from build123d import *

# Parameters (mm, degrees)
SKETCH1_R          = 10
SKETCH1_R_2        = 2.5
SKETCH1_R_3        = 15
SKETCH1_R_4        = 5
BASE_FLANGE1_DEPTH = 3.4


# Sheet-metal steps are written as plain solids
with BuildPart() as part:
    # Sketch1 → Base-Flange1 (new body)
    with BuildSketch(Plane.XY):
        Polygon((0, 63.731432889), (0, 0), (-95.246303627, 0), (-424.746303627, 118), (-484.746303627, 118), (-594.746303627, 58), (-654.746303627, 58), (-654.746303627, 118), (-594.746303627, 118), (-484.746303627, 181.731432889), (-424.746303627, 181.731432889), (-95.246303627, 63.731432889), align=None)
        with Locations((-624.746303627, 88)):
            Circle(SKETCH1_R, mode=Mode.SUBTRACT)
        with Locations((-454.746303627, 149.865716445)):
            Circle(SKETCH1_R, mode=Mode.SUBTRACT)
        with Locations((-539.746303627, 118.932858222)):
            Circle(SKETCH1_R_2, mode=Mode.SUBTRACT)
        with Locations((-161.147850314, 55.466270342)):
            Circle(SKETCH1_R_3, mode=Mode.SUBTRACT)
        with Locations((-255.29291701, 89.181347338)):
            Circle(SKETCH1_R_2, mode=Mode.SUBTRACT)
        with Locations((-349.437983706, 122.896424333)):
            Circle(SKETCH1_R_3, mode=Mode.SUBTRACT)
        with Locations((-429.746303627, 149.865716445)):
            Circle(SKETCH1_R_2, mode=Mode.SUBTRACT)
        with Locations((-479.746303627, 149.865716445)):
            Circle(SKETCH1_R_2, mode=Mode.SUBTRACT)
        with Locations((-60.9, 12.7)):
            Circle(SKETCH1_R_4, mode=Mode.SUBTRACT)
        with Locations((-95.246303627, 46.865716445)):
            Circle(SKETCH1_R_2, mode=Mode.SUBTRACT)
        with Locations(Location((-9.1, 12.7, 0), (0, 0, 180))):
            Circle(SKETCH1_R_4, mode=Mode.SUBTRACT)
    extrude(amount=-BASE_FLANGE1_DEPTH)


solid = part.part
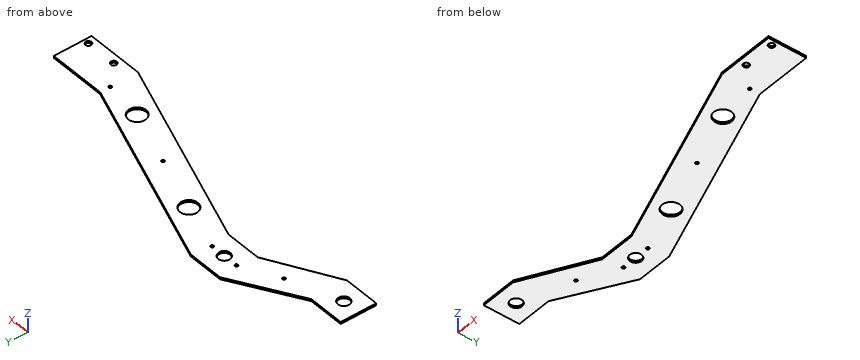
Geometry check sheet. Reference: the model listing, model coordinates, mm. Round coordinates to 2 decimals unless told otherwise and drop trailing zeros. Write each loop counter-clockwise with the first axis right and the second up, starting at its lowest first coordinate (ties: lowest second). Pieces come first, ordered by that corner, then holes.
Item 1: Section check A-A (x = -458). Record the boundary of the cut face in (y, z), plus the area to 3 significant figures.
Determined:
outline: (118, -3.4) - (140.41, -3.4) - (140.41, 0) - (118, 0) - close; (159.32, -3.4) - (181.73, -3.4) - (181.73, 0) - (159.32, 0) - close
area: 152 mm2
Item 2: Material ranges on line 1 along Y through (x, z) = (-60.9, -2.55); line 2 along Y through (x, z) = (-469, -3); line 3 along Y through (x, z) = (-502.5, -1.1), recorded low to high.
Determined:
line 1: y = 0 to 7.7, 17.7 to 63.73
line 2: y = 118 to 181.73
line 3: y = 108.32 to 171.45
Item 3: Go/stop test with flat-tipped pins: pin 1 Ø1 at (x, z) = (-95.5, -0.5) entering from +Y; pin 2 Ø13 at (x, y) = (-60.9, 12.7) entering from +Z; pin 3 Ø1.7 at (x, z) = (-56.5, -1) entering from +Y; pin 4 Ø1.5 at (x, z) = (-269.5, -3) entering from -Y. Record where each tip stops, or that it passes through.
Determined:
pin 1: stops at y = 64
pin 2: stops at z = 0
pin 3: stops at y = 63.73
pin 4: stops at y = 62.13
Item 4: Section check D-D (x = -548). Record the boundary of the cut face in (y, z), plus the area to 3 significant figures.
Determined:
outline: (83.5, -3.4) - (145.08, -3.4) - (145.08, 0) - (83.5, 0) - close
area: 209 mm2
Item 5: Section check C-C (y = 25). Record the boundary of the cut face in (x, z).
Determined:
outline: (-165.06, -3.4) - (0, -3.4) - (0, 0) - (-165.06, 0) - close
Item 6: Section check B-B (z = -1.9). Give the number of separate pieces and of enclosed holes in the cut face, plus the area to 3 significant figures.
Determined:
separate pieces: 1
enclosed holes: 11
area: 39,000 mm2
